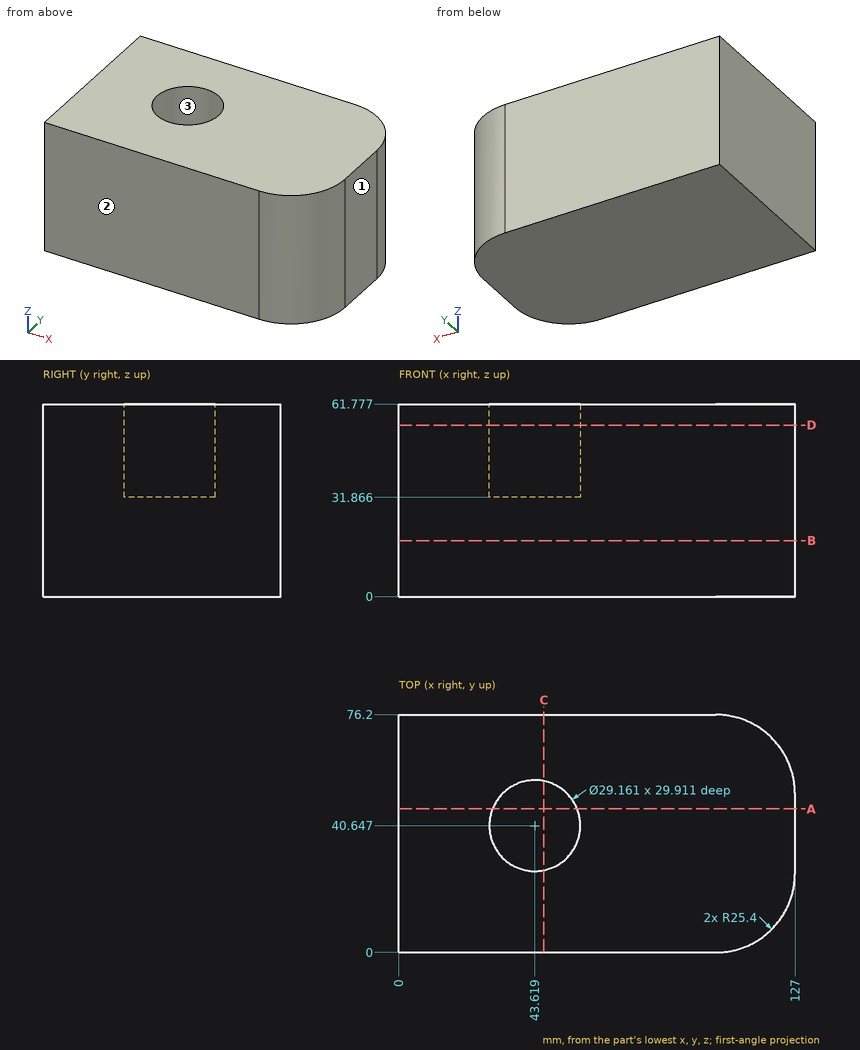
Print and shaded views of the part. All mm, measured from the part's lowest x, y and z. Give positions to 0.01 mm unless a question says otherwise; leave off trailing zeros. Loops run counter-clockwise (first coordinate to the right, second up) from the corner with the lowest first, then second, coordinate; pieces in that order, holes last.
1) Saw through at D-D (z = 55). Write the cut outline in (x, y).
2) Saw through at A-A (y = 46). Write the cut outline in (x, z).
3) Wall check: line 1 (Y direction, x = 44, z = 58.5); line 2 (Z direction, x = 42.5, y = 37); line 3 (X direction, y = 45, z = 55.5) (1 decimal). Give the ranges that are in metal, low to high.
4) Flat gauge pins, fed straight in: pin 1 Ø23.5 at (x, y) = (43.62, 40.65) entering from +Z; pin 2 Ø1.5 at (y, z) = (67.5, 55.5) entering from +X; pin 3 Ø2 at (y, z) = (64, 39.5) entering from +X. Where does each tip first touch, or does it go through?
5) Pull direction Y, two halves, no side cores. Call the marked faces 1, 2 and 3: +Y half, -Y half, draft (parallel to the pull), parting line (faces both ways), or undercut.
6) Saw through at B-B (z = 18). Write the cut outline in (x, y), plus the area to 3 significant figures.
7) Saw through at C-C (x = 46.5). Write the cut outline in (y, z), plus the area to 3 significant figures.
Answer block:
1. outline: (0, 0) - (101.6, 0) arc R25.4 ccw to (127, 25.4) - (127, 50.8) arc R25.4 ccw to (101.6, 76.2) - (0, 76.2) - close; hole circle Ø29.16 at (43.62, 40.65)
2. outline: (0, 0) - (127, 0) - (127, 61.78) - (57.18, 61.78) - (57.18, 31.87) - (30.06, 31.87) - (30.06, 61.78) - (0, 61.78) - close
3. line 1: y = 0 to 26.07, 55.22 to 76.2
3. line 2: z = 0 to 31.87
3. line 3: x = 0 to 29.7, 57.5 to 127
4. pin 1: stops at z = 31.87
4. pin 2: stops at x = 121.37
4. pin 3: stops at x = 123.88
5. face 1: draft
5. face 2: -Y half
5. face 3: undercut
6. outline: (0, 0) - (101.6, 0) arc R25.4 ccw to (127, 25.4) - (127, 50.8) arc R25.4 ccw to (101.6, 76.2) - (0, 76.2) - close
6. area: 9,400 mm2
7. outline: (0, 0) - (76.2, 0) - (76.2, 61.78) - (54.94, 61.78) - (54.94, 31.87) - (26.35, 31.87) - (26.35, 61.78) - (0, 61.78) - close
7. area: 3,850 mm2
